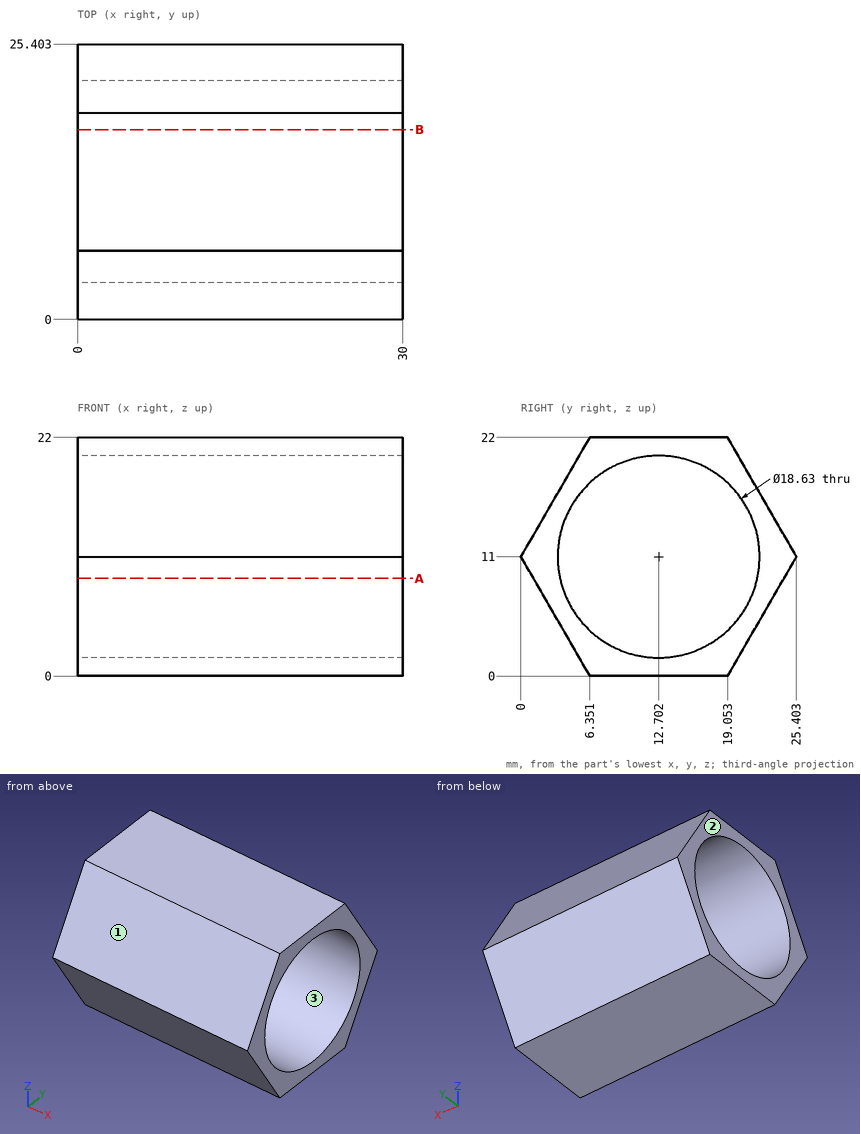
Job drawing, mm, ordinate dimensions from the low corner. One solid piece. Give positions to 0.01 mm unless a question says otherwise; leave off trailing zeros. Write each loop counter-clockwise with the first axis right and the second up, starting at its lowest first coordinate (ties: lowest second). Pieces come first, ordered by that corner, then holes. Notation, with made-up numbers: (-3.75, 19) - (34.25, 19) arc R31 ccw to (34.25, 51) - close; hole circle Ø4 at (-36.75, 25.5). An arc over 180 degrees is marked (long way). Use one line per item in the form item = value. Start each with the question number.
1. Drop flat-ended pins along their axis: pin 1 Ø10 at (x, z) = (15.5, 3) entering from +Y; pin 2 Ø5 at (x, z) = (19, 17.5) entering from +Y (1 decimal); pin 3 Ø2 at (x, z) = (15, 8) entering from -Y (1 decimal); pin 4 Ø5 at (y, z) = (13, 16) entering from -X. Give the stop position or say it passes through.
2. Two-plate mould, pull along Y, no slides. Class the marked faces 1, 2 and 3: released by +Y, released by -Y, zero draft, split by the parting line, or undercut.
3. Probe line 1 (Y direction, x = 26, z = 5.5) (1 decimal); line 2 (Y direction, x = 15, z = 13.5) (1 decimal); line 3 (Z direction, x = 6, y = 16.25). List the from-to ranges inside material, lowest first. Write a range as [from, to].
4. Band-saw the part on A-A on z = 9. Write the cut outline in (x, y) (1 decimal), plus the area to 3 significant figures.
5. Band-saw the part on B-B on y = 17.5. Write the cut outline in (x, z).
Conclusion:
q1.pin_1 = 23.67
q1.pin_2 = 23.1
q1.pin_3 = 1.2
q1.pin_4 = through
q2.face_1 = released by -Y
q2.face_2 = zero draft
q2.face_3 = undercut
q3.line_1 = [3.2, 5.2], [20.2, 22.2]
q3.line_2 = [1.4, 3.7], [21.7, 24]
q3.line_3 = [0, 2.39], [19.61, 22]
q4.outline = (0, 1.2) - (30, 1.2) - (30, 3.6) - (0, 3.6) - close; (0, 21.8) - (30, 21.8) - (30, 24.2) - (0, 24.2) - close
q4.area = 147 mm²
q5.outline = (0, 0) - (30, 0) - (30, 3.02) - (0, 3.02) - close; (0, 18.98) - (30, 18.98) - (30, 22) - (0, 22) - close
